from build123d import *

# Parameters (mm, degrees)
F1_R     = 9
F1_R_2   = 3.5
F2_DEPTH = 2
F0_R     = 3.5
F0_R_2   = 2.5
F4_DEPTH = 3
F5_R     = 2.5
F3_R     = 2.5
F6_DEPTH = 5


with BuildPart() as f2:
    # F1 (on face) → F2 (new body)
    with BuildSketch(Plane.XY):
        Circle(F1_R)
        Circle(F1_R_2, mode=Mode.SUBTRACT)
    extrude(amount=F2_DEPTH)

    # F0 (on Top) → F4 (join)
    with BuildSketch(Plane.XY):
        Circle(F0_R)
        Circle(F0_R_2, mode=Mode.SUBTRACT)
    extrude(amount=F4_DEPTH)

    # F5 (on Top) + F3 (on face) → F6 (join)
    with BuildSketch(Plane.XY):
        Circle(F5_R)
    with BuildSketch(Plane.XY):
        Circle(F3_R)
    extrude(amount=F6_DEPTH)


solid = f2.part
Geometry check sheet. Reference: the model listing, model coordinates, mm. A direction names the side the tool comes from. Give positions to 0.01 mm unless a question says otherwise; leave off trailing zeros. Order: outer loops, then holes, each group sorted by start corner. A loop starts at its lowest first (then second) coordinate and runs counter-clockwise, first axis right, second up. Notation, with made-up numbers: (20.25, 86) - (69.25, 86) arc R21 cw to (69.25, 102) - close; hole circle Ø5 at (81.25, 70.25). An arc over 180 degrees is marked (long way). Answer as a JSON object with one key per item and string values.
(1) Cross-section at D-D (y = -3). Record the cut outline in (x, z), then the cut area to 3 significant figures.
Report:
{"outline": "(-8.49, 0) - (8.49, 0) - (8.49, 2) - (1.8, 2) - (1.8, 3) - (-1.8, 3) - (-1.8, 2) - (-8.49, 2) - close", "area": "37.5 mm^2"}
(2) Tool access check on faces 1 (the cylindrical face through (-1.172, 8.923, 0.986)), 2 (the cylindrical face through (3.233, -1.341, 2.493)). Record the directions out of +Z, -Z, +X, -X, +Y, -Y that give a thin tool (end or side, any length) a straight path to the whole face; none if there is none.
Report:
{"face 1": "+Z, -Z", "face 2": "+Z"}
(3) Depth check by flat-ended pin: pin 1 Ø1 at (y, z) = (-7, 1.5) entering from -X; pin 2 Ø2 at (x, y) = (5.5, -1.5) entering from -Z; pin 3 Ø2 at (x, z) = (5, 4) entering from +Y; pin 4 Ø3 at (y, z) = (4, 1) entering from +X. Enter the tip coordinate at first touch or a pass-through.
Report:
{"pin 1": "x = -6.22", "pin 2": "z = 0", "pin 3": "through", "pin 4": "x = 8.65"}
(4) Cross-section at C-C (z = 2.5). Record the cut outline in (x, y), then the cut area to 3 significant figures.
Report:
{"outline": "circle Ø7 at (0, 0)", "area": "38.5 mm^2"}
(5) Cross-section at A-A (y = 0). Record the cut outline in (x, z), then the cut area to 3 significant figures.
Report:
{"outline": "(-9, 0) - (9, 0) - (9, 2) - (3.5, 2) - (3.5, 3) - (2.5, 3) - (2.5, 5) - (-2.5, 5) - (-2.5, 3) - (-3.5, 3) - (-3.5, 2) - (-9, 2) - close", "area": "53.0 mm^2"}
(6) Material ranges on line 1 (Z direction, x = -6, y = -5.25); line 2 (Z direction, x = -1.75, y = 2); line 3 (Y direction, x = 2.5, z = 2.35), recorded low to high.
Report:
{"line 1": "0 to 2", "line 2": "0 to 3", "line 3": "-2.45 to 2.45"}
